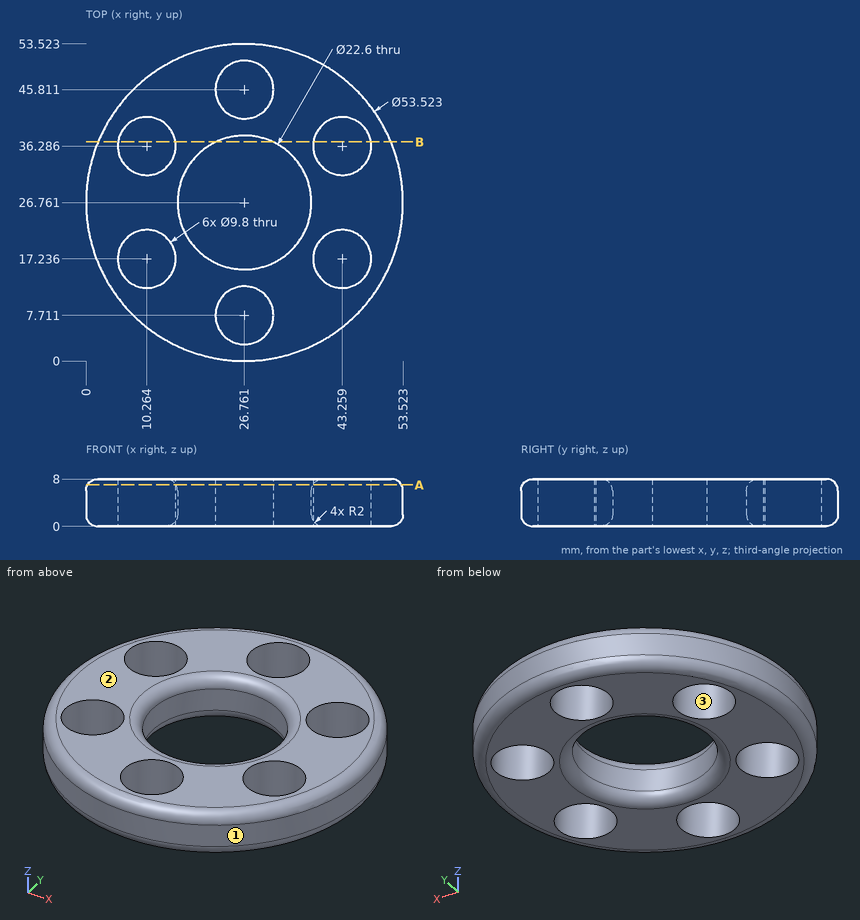
Print and shaded views of the part. All mm, measured from the part's lowest x, y and z. Round coordinates to 2 decimals unless told otherwise and drop trailing zeros. Write each loop counter-clockwise with the first axis right and the second up, starting at its lowest first coordinate (ties: lowest second). Pieces come first, ordered by that corner, then holes. Notation, with made-up numbers: (-20.5, 20) -> (29.5, 20) arc R29 cw to (29.5, 47) -> close; hole circle Ø10 at (69.25, 46). An arc over 180 degrees is marked (long way). Write item = value, one per line.
(1) Probe L1, parallel to Y at x = 12.5, z = 7 (1 decimal); L2, parallel to Y at x = 40, z = 0.5 (1 decimal); L3, parallel to Y at x = 35, z = 7.5 (1 decimal). List the from-to ranges inside material, lowest first.
Answer:
L1 = 4.4 to 12.9, 21.6 to 31.9, 40.6 to 49.1
L2 = 4.3 to 13.6, 20.9 to 32.6, 39.9 to 49.2
L3 = 2 to 18.1, 35.5 to 51.5
(2) Band-saw the part on A-A (z = 7). Give the cut face in (x, y) (1 decimal).
Answer:
outline = circle Ø53 at (26.8, 26.8); hole circle Ø9.8 at (10.3, 17.2); hole circle Ø9.8 at (10.3, 36.3); hole circle Ø23.1 at (26.8, 26.8); hole circle Ø9.8 at (26.8, 7.7); hole circle Ø9.8 at (26.8, 45.8); hole circle Ø9.8 at (43.3, 17.2); hole circle Ø9.8 at (43.3, 36.3)
(3) Flat gauge pins, fed straight in: pin 1 (4 mm diameter, centred on x = 41, z = 5.5, fed in from -Y); pin 2 (1.5 mm diameter, centred on x = 30, z = 2.5, fed in from +Y); pin 3 (3 mm diameter, centred on x = 21, z = 4.5, fed in from +Y). Where does each tip first touch, or does it go through?
Answer:
pin_1 = 2.96
pin_2 = 53.41
pin_3 = 53.18
(4) Band-saw the part on B-B (y = 37). State how many separate pieces and enclosed holes the cut face has, then the cut area to 3 significant figures.
Answer:
separate_pieces = 4
enclosed_holes = 0
area = 153 mm2
(5) Two-plate mould, pull along X, no slides. Class the marked faces 1, 2 and 3: pulls with the +X half, pulls with the -X half, needs draft (parallel to the pull), parting line crosses it, or undercut.
Answer:
face_1 = parting line crosses it
face_2 = needs draft
face_3 = undercut
